For this review, take the finished solid that the model builds, in its own axes (mm). Round coordinates to 2 decimals unless told otherwise and drop trailing zeros. Answer as CSV lines item,"result". Start each with the question number.
Item 1: For pin 1 Ø5 at (y, z) = (288, -1.5) entering from +X; pin 2 Ø13 at (x, y) = (-20, 529) entering from -Z; pin 3 Ø8 at (y, z) = (110, -0.5) entering from -X, all flat-tipped, find the tip position at first contact; note any pin that passes through.
Item 2: Take a section at A-A on y = 630. Count the separate pieces of the cut face and the enclosed holes in it, then the cut area to 3 significant figures.
Item 3: Wall thickness on probe 1 along X at (y, z) = (238.5, 14.5); probe 2 along X at (y, z) = (46.5, 5.5); probe 3 along X at (y, z) = (293, -1): over which ranges is each line inside the solid? List them lowest first. Write a range as from..to.
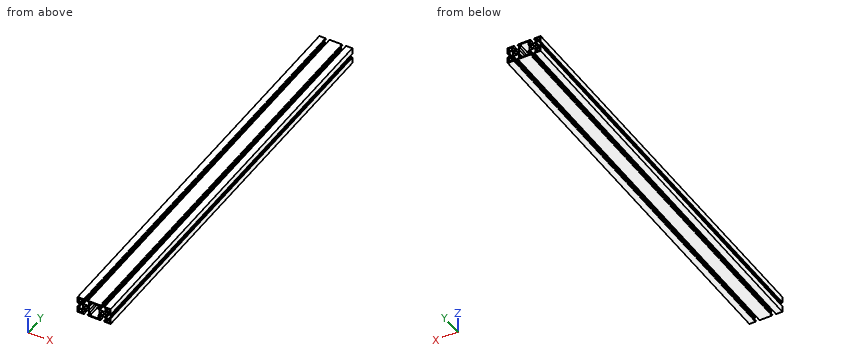
```python
from build123d import *

# Parameters (mm, degrees)
SKETCH1_W           = 80
SKETCH1_H           = 40
BOSS_EXTRUDE1_DEPTH = 1000
SKETCH2_W           = 7.8
SKETCH2_H           = 7.8
CUT_EXTRUDE1_DEPTH  = 1001
SKETCH3_R           = 3.5
CUT_EXTRUDE2_DEPTH  = 1001


with BuildPart() as part:
    # Sketch1 → Boss-Extrude1 (new body)
    with BuildSketch(Plane(origin=(0, 0, 0), x_dir=(1, 0, 0), z_dir=(0, 1, 0))):
        Rectangle(SKETCH1_W, SKETCH1_H)
        Polygon((-27.8, -17.8), (-12.2, -17.8), (-12.2, -8.925), (-14.125, -7), (-25.875, -7), (-27.8, -8.925), align=None, mode=Mode.SUBTRACT)
        Polygon((-28.925, -7.8), (-37.8, -7.8), (-37.8, 7.8), (-28.925, 7.8), (-27, 5.875), (-27, -5.875), align=None, mode=Mode.SUBTRACT)
        Polygon((-27.8, 8.925), (-27.8, 17.8), (-12.2, 17.8), (-12.2, 8.925), (-14.125, 7), (-25.875, 7), align=None, mode=Mode.SUBTRACT)
        Polygon((27.8, 17.8), (12.2, 17.8), (12.2, 8.925), (14.125, 7), (25.875, 7), (27.8, 8.925), align=None, mode=Mode.SUBTRACT)
        Polygon((37.8, -7.8), (37.8, 7.8), (28.925, 7.8), (27, 5.875), (27, -5.875), (28.925, -7.8), align=None, mode=Mode.SUBTRACT)
        Polygon((27.8, -8.925), (27.8, -17.8), (12.2, -17.8), (12.2, -8.925), (14.125, -7), (25.875, -7), align=None, mode=Mode.SUBTRACT)
    extrude(amount=BOSS_EXTRUDE1_DEPTH)

    # Sketch2 → Cut-Extrude1 (cut, through all)
    with BuildSketch(Plane(origin=(0, 1000, 0), x_dir=(1, 0, 0), z_dir=(0, 1, 0))):
        with Locations((33.9, -13.9)):
            Rectangle(SKETCH2_W, SKETCH2_H)
        Polygon((-10, -17.8), (-10, -8.875), (-13, -5.875), (-13, 5.875), (-10, 8.875), (-10, 17.8), (10, 17.8), (10, 8.875), (13, 5.875), (13, -5.875), (10, -8.875), (10, -17.8), align=None)
        with Locations((33.9, 13.9)):
            Rectangle(SKETCH2_W, SKETCH2_H)
        with Locations((-33.9, -13.9)):
            Rectangle(SKETCH2_W, SKETCH2_H)
        with Locations((-33.9, 13.9)):
            Rectangle(SKETCH2_W, SKETCH2_H)
    extrude(amount=-CUT_EXTRUDE1_DEPTH, mode=Mode.SUBTRACT)

    # Sketch3 → Cut-Extrude2 (cut, through all)
    with BuildSketch(Plane(origin=(0, 1000, 0), x_dir=(1, 0, 0), z_dir=(0, 1, 0))):
        with Locations((-20, 0)):
            Circle(SKETCH3_R)
        with Locations((20, 0)):
            Circle(SKETCH3_R)
        Polygon((-25.1, 20), (-25.1, 18.9), (-24.1, 18.9), (-24.1, 17.8), (-15.9, 17.8), (-15.9, 18.9), (-14.9, 18.9), (-14.9, 20), align=None)
        Polygon((-37.8, 4.1), (-37.8, -4.1), (-38.9, -4.1), (-38.9, -5.1), (-40, -5.1), (-40, 5.1), (-38.9, 5.1), (-38.9, 4.1), align=None)
        Polygon((-24.1, -17.8), (-15.9, -17.8), (-15.9, -18.9), (-14.9, -18.9), (-14.9, -20), (-25.1, -20), (-25.1, -18.9), (-24.1, -18.9), align=None)
        Polygon((25.1, -20), (25.1, -18.9), (24.1, -18.9), (24.1, -17.8), (15.9, -17.8), (15.9, -18.9), (14.9, -18.9), (14.9, -20), align=None)
        Polygon((40, 5.1), (38.9, 5.1), (38.9, 4.1), (37.8, 4.1), (37.8, -4.1), (38.9, -4.1), (38.9, -5.1), (40, -5.1), align=None)
        Polygon((24.1, 17.8), (15.9, 17.8), (15.9, 18.9), (14.9, 18.9), (14.9, 20), (25.1, 20), (25.1, 18.9), (24.1, 18.9), align=None)
    extrude(amount=-CUT_EXTRUDE2_DEPTH, mode=Mode.SUBTRACT)


solid = part.part
```
Output values:
1,pin 1,"stops at x = 27"
1,pin 2,"stops at z = -20"
1,pin 3,"stops at x = -38.9"
2,separate pieces,"1"
2,enclosed holes,"7"
2,area,"969 mm^2"
3,probe 1,"x = -40..-37.8, -30..-27.8, -12.2..-10, 10..12.2, 27.8..30, 37.8..40"
3,probe 2,"x = -40..-37.8, -27..-13, 13..27, 37.8..40"
3,probe 3,"x = -27..-23.35, -16.65..-13, 13..16.65, 23.35..27"
